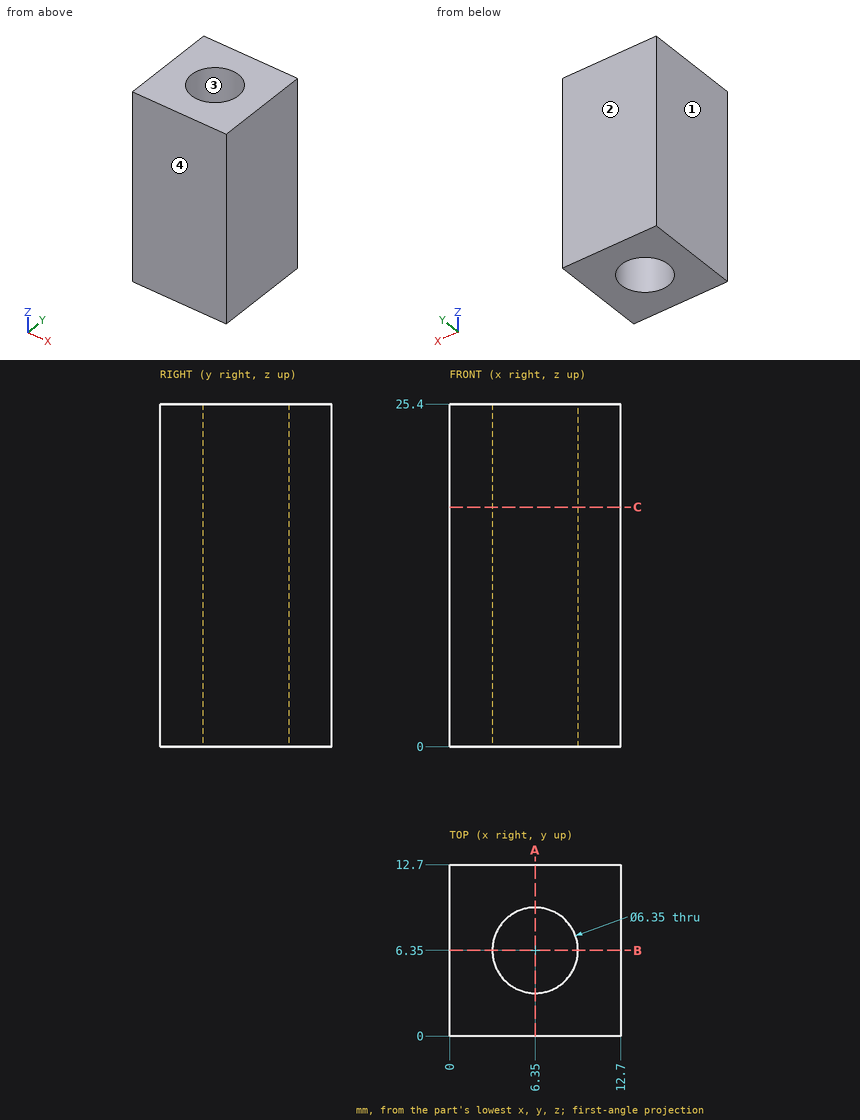
Check sheet for the drawn part. Datum: minimum x, y, z corner. Units: mm. Round coordinates to 2 decimals unless told otherwise and drop trailing zeros. Order: outer loops, then holes, each group sorted by start corner. A loop starts at its lowest first (then second) coordinate and runs counter-clockwise, first axis right, second up. Notation, with made-up numbers: (11, 81) - (26, 81) arc R10 ccw to (26, 87) - close; hole circle Ø5 at (38, 12). An arc over 180 degrees is marked (long way). Use a Markdown table: item, result. Add a question column.
(1) Material ranges on line 1 along Y through (x, z) = (6.35, 15) (3 decimals); line 2 along Y through (x, z) = (5.5, 8); line 3 along X through (y, z) = (3.5, 3.25), recorded low to high. Write a range as [from, to].
(2) Release check for a two-part mould opening along Y. For the marked faces 1, 2, 3 and 4 record: pulls with the +Y half, pulls with the -Y half, needs draft (parallel to the pull), parting line crosses it, or undercut.
(3) Depth check by flat-ended pin: pin 1 (5.5 mm diameter, centred on x = 6.35, y = 6.35, fed in from +Z). Enter the tip coordinate at first touch or a pass-through.
(4) Sectioned sample at A-A, the plane x = 6.35. Enter the section's corners in (y, z) (3 decimals), and give its area (3 significant figures).
(5) Sectioned sample at C-C, the plane z = 17.75. Enter the section's corners in (x, y) (3 decimals).
Answers below:
| question | item | result |
|---|---|---|
| 1 | line 1 | [0, 3.175], [9.525, 12.7] |
| 1 | line 2 | [0, 3.29], [9.41, 12.7] |
| 1 | line 3 | [0, 4.95], [7.75, 12.7] |
| 2 | face 1 | needs draft |
| 2 | face 2 | pulls with the +Y half |
| 2 | face 3 | undercut |
| 2 | face 4 | pulls with the -Y half |
| 3 | pin 1 | through |
| 4 | outline | (0, 0) - (3.175, 0) - (3.175, 25.4) - (0, 25.4) - close; (9.525, 0) - (12.7, 0) - (12.7, 25.4) - (9.525, 25.4) - close |
| 4 | area | 161 mm² |
| 5 | outline | (0, 0) - (12.7, 0) - (12.7, 12.7) - (0, 12.7) - close; hole circle Ø6.35 at (6.35, 6.35) |
